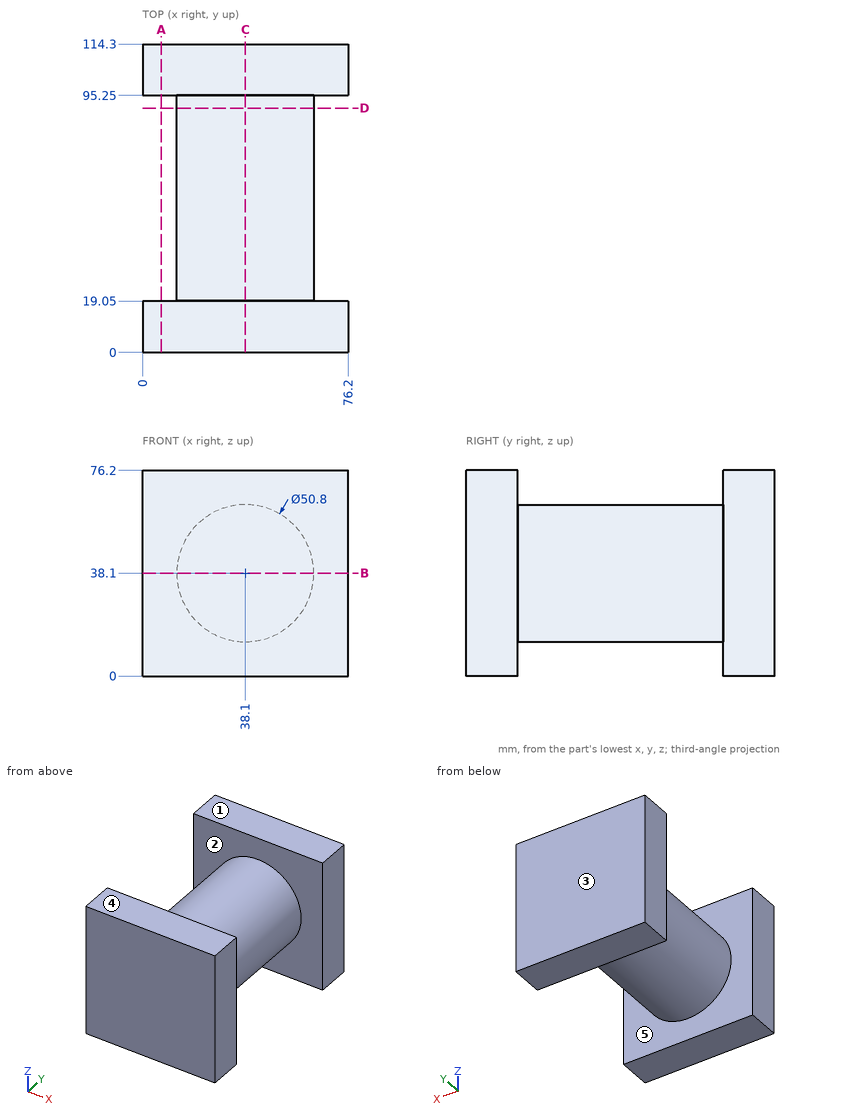
Check sheet for the drawn part. Datum: minimum x, y, z corner. Units: mm. A direction names the side the tool comes from. Round coordinates to 2 decimals unless told otherwise and drop trailing zeros. Write each loop counter-clockwise with the first axis right and the second up, starting at its lowest first coordinate (ties: lowest second). Pieces come first, ordered by that corner, then holes. Notation, with made-up numbers: (88.5, 35.25) -> (115.5, 35.25) arc R17 ccw to (115.5, 51.25) -> close; hole circle Ø1 at (65.25, -0.75). An arc over 180 degrees is marked (long way). One line per item, written item: value. Start each with the question number.
(1) Scan lines: line 1 (Y direction, x = 17, z = 54); line 2 (Z direction, x = 45, y = 66.5). Record each from-to range of solid material in increasing order. Write a range as [from, to].
(2) Cross-section at B-B, the plane z = 38.1. Record the cut outline in (x, y).
(3) Draft check along Y on the marked faces 1, 2 and 3. Enter one of: +Y half, -Y half, draft (parallel to the pull), parting line (faces both ways), or undercut.
(4) Go/stop test with flat-tipped pins: pin 1 Ø4 at (x, z) = (23.5, 40) entering from -Y; pin 2 Ø4 at (y, z) = (42.5, 63) entering from -X; pin 3 Ø12 at (x, y) = (38.5, 33.5) entering from -Z; pin 4 Ø5 at (y, z) = (72.5, 13.5) entering from +X. Record where each tip stops, or that it passes through.
(5) Cross-section at A-A, the plane x = 7. Record the cut outline in (y, z), and give its area (3 significant figures).
(6) Cross-section at C-C, the plane x = 38.1. Record the cut outline in (y, z), and give its area (3 significant figures).
(7) Access from +Z, -Z, +X, -X, +Y, -Y to the whole of each face (thin tool, end or side, straight path). Record for the marked faces 4 and 5.
(8) Cross-section at D-D, the plane y = 90.5. Record the cut outline in (x, z).
Answer:
1. line 1: [0, 19.05], [95.25, 114.3]
1. line 2: [13.66, 62.54]
2. outline: (0, 0) -> (76.2, 0) -> (76.2, 19.05) -> (63.5, 19.05) -> (63.5, 95.25) -> (76.2, 95.25) -> (76.2, 114.3) -> (0, 114.3) -> (0, 95.25) -> (12.7, 95.25) -> (12.7, 19.05) -> (0, 19.05) -> close
3. face 1: draft
3. face 2: undercut
3. face 3: +Y half
4. pin 1: y = 0
4. pin 2: x = 27.11
4. pin 3: z = 12.7
4. pin 4: x = 50.62
5. outline: (0, 0) -> (19.05, 0) -> (19.05, 76.2) -> (0, 76.2) -> close; (95.25, 0) -> (114.3, 0) -> (114.3, 76.2) -> (95.25, 76.2) -> close
5. area: 2,900 mm²
6. outline: (0, 0) -> (19.05, 0) -> (19.05, 12.7) -> (95.25, 12.7) -> (95.25, 0) -> (114.3, 0) -> (114.3, 76.2) -> (95.25, 76.2) -> (95.25, 63.5) -> (19.05, 63.5) -> (19.05, 76.2) -> (0, 76.2) -> close
6. area: 6,770 mm²
7. face 4: +Z, +X, -X, +Y, -Y
7. face 5: none
8. outline: circle Ø50.8 at (38.1, 38.1)
